Source: three-view drawing plus pictorial views. Frame: mm from the lowest corner of the part. A direction names the side the tool comes from. Round coordinates to 2 decimals unless told otherwise and drop trailing zeros. Loops run counter-clockwise (first coordinate to the right, second up) from the corner with the lowest first, then second, coordinate; pieces in that order, holes last. Notation, with made-up numbers: M 50.25,-1 L 108.25,-1 A14 cw 108.25,7 Z; hole C -26,-5.75 d2. An arc over 180 degrees is marked long. Write each question's results on one line, items separated by ' | '.
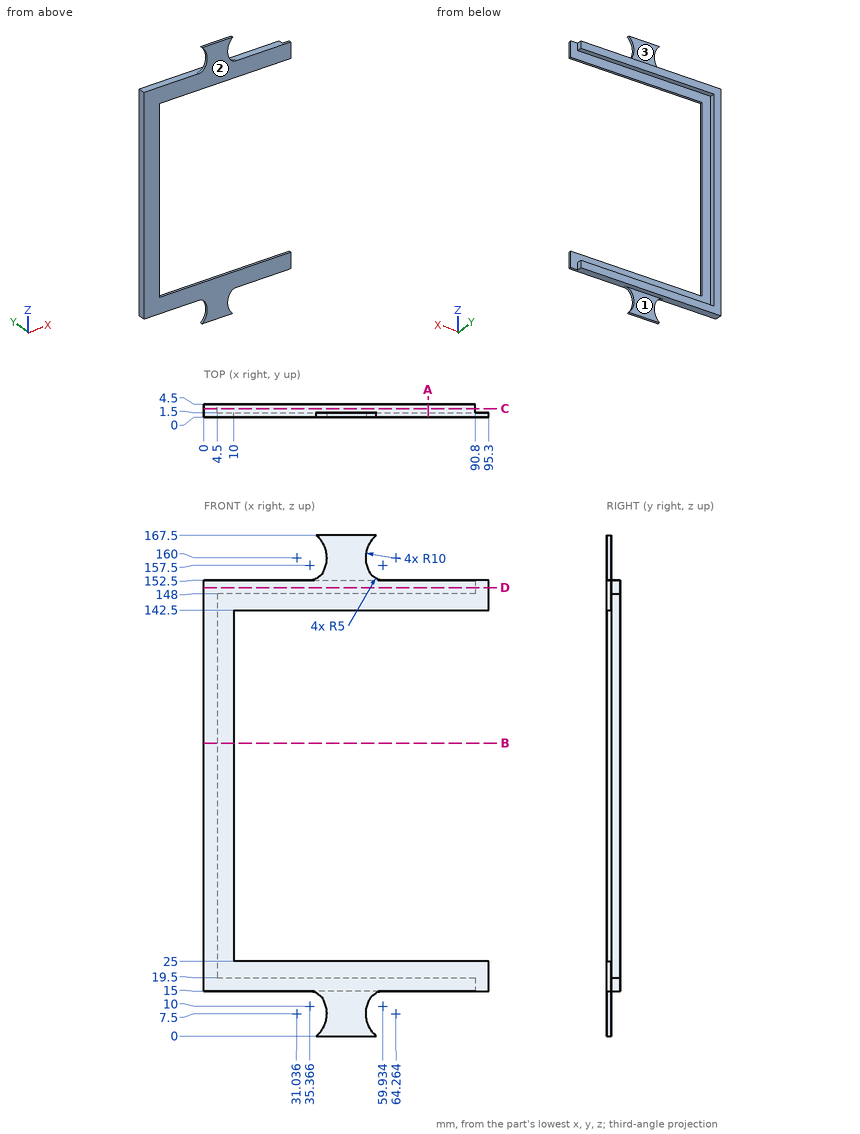
1. Section D-D (z = 150). Output: boundary loops of the cut face in (x, y).
Answer key:
outline: M 0,0 L 95.3,0 L 95.3,1.5 L 90.8,1.5 L 90.8,4.5 L 0,4.5 Z
2. Section C-C (y = 2.95). Output: boundary loops of the cut face in (x, z).
Answer key:
outline: M 0,15 L 90.8,15 L 90.8,19.5 L 4.5,19.5 L 4.5,148 L 90.8,148 L 90.8,152.5 L 0,152.5 Z
3. Section B-B (z = 98). Output: boundary loops of the cut face in (x, y).
Answer key:
outline: M 0,0 L 10,0 L 10,1.5 L 4.5,1.5 L 4.5,4.5 L 0,4.5 Z
4. Ray query, probe 1 along Z at (x, y) = (67, 4.1); probe 2 along Z at (x, y) = (26, 1.45); probe 3 along X at (y, z) = (0.8, 89.5). Return the intervals inside material, ascending.
Answer key:
probe 1: z = 15 to 19.5, 148 to 152.5 | probe 2: z = 15 to 25, 142.5 to 152.5 | probe 3: x = 0 to 10
5. Pin query (flat end, axial travel): P1, Ø1.5, axis at x = 27, y = 2.5, coming from the -Z side; P2, Ø2, axis at x = 67.5, y = 0.5, coming from the +Z side; P3, Ø7.5, axis at x = 43, z = 9, coming from the +Y side. Return the tip coordinate at first contact, or that it passes through.
Answer key:
P1: stops at z = 15 | P2: stops at z = 152.5 | P3: stops at y = 1.5
6. Section A-A (x = 75). Output: boundary loops of the cut face in (y, z).
Answer key:
outline: M 0,15 L 4.5,15 L 4.5,19.5 L 1.5,19.5 L 1.5,25 L 0,25 Z; M 0,142.5 L 1.5,142.5 L 1.5,148 L 4.5,148 L 4.5,152.5 L 0,152.5 Z
7. Access query for the marked faces 1, 2 and 3. Directions: +Z, -Z, +X, -X, +Y, -Y. A direction counts if a zero-diameter tool reaches every point of the face in a straight line with its end or side. Return the directions, or none.
Answer key:
face 1: -Z, +X, -X, +Y | face 2: +Z, -Z, +X, -X, -Y | face 3: +Z, +X, -X, +Y
